Read the model definition and answer for the solid it produces. Units are mm, in the model's axes. Coordinates: 2 decimals unless noted, no trailing zeros. Loops run counter-clockwise (first coordinate to the right, second up) from the corner with the lowest first, then second, coordinate; pieces in that order, holes last. Notation, with made-up numbers: (29.25, -8) -> (70.25, -8) arc R23 cw to (70.25, 1) -> close; hole circle Ø9 at (50, 69.25). An arc over 180 degrees is marked (long way). Answer as a JSON object with one key per item and string values. Group by question number.
1) Section B-B, the plane y = 0 is taken. Give the vertices of the cut face in (x, z), plus the area to 3 significant figures.
2) Section D-D, the plane y = -37.7 is taken. Give the vertices of the cut face in (x, z).
3) Consider probe 1 along X at (y, z) = (0.5, 8.75); probe 2 along Y at (x, z) = (0, 7.25); probe 3 along Y at (x, z) = (17, 2.75). Determine where each line is inside the solid, lowest interval first. Write a range as [from, to].
4) Section A-A, the plane z = 8 is taken. Count the separate pieces of the cut face and the enclosed holes in it, plus the area to 3 significant figures.
5) Determine the mould class of faces 1 (the face through (36.325, -18.426, 4.93)), 2 (the face through (31.4, -18.8, 5.1)), 3 (the face through (-1, 1, 0)) for opening direction Y: released by +Y, released by -Y, zero draft, split by the parting line, or undercut.
6) Flat-ended cylindrical pins translate along their axes: P1, Ø3, axis at y = 10.5, z = 7, coming from the +X side; P2, Ø0.5, axis at x = 38.5, z = 3.5, coming from the -Y side; P3, Ø1.5, axis at y = -23.5, z = 6.5, coming from the -X side; P4, Ø2, axis at x = -32.65, y = -18.85, coming from the +Z side. Find the tip coordinate at first contact, or state that the pin passes through.
7) Section C-C, the plane x = 15 is taken. Give the vertices of the cut face in (y, z).
from build123d import *

# Parameters (mm, degrees)
SKETCH_1_R          = 45.3
EXTRUDE_1_DEPTH     = 10
CUT_EXTRUDE_1_DEPTH = 11
FILLET_1_R          = 3
SKETCH_3_R          = 1.25
CUT_EXTRUDE_2_DEPTH = 11
SKETCH_4_R          = 5.1
CUT_EXTRUDE_3_DEPTH = 11


with BuildPart() as part:
    # 草图1 → 凸台-拉伸1 (new body)
    with BuildSketch(Plane.XY):
        Circle(SKETCH_1_R)
    extrude(amount=EXTRUDE_1_DEPTH)

    # 草图2 → 切除-拉伸1 (cut, through all)
    with BuildSketch(Plane.XY.offset(10)):
        with BuildLine():
            Line((-36.056760808, 18), (-41.570301899, 18))
            ThreePointArc((-41.570301899, 18), (0, 45.3), (41.570301899, 18))
            Line((41.570301899, 18), (36.056760808, 18))
            ThreePointArc((36.056760808, 18), (0, 40.3), (-36.056760808, 18))
        make_face()
        with BuildLine():
            Line((-36.056760808, -18), (-41.734622438, -18))
            ThreePointArc((-41.734622438, -18), (0, -45.450838386), (41.734622438, -18))
            Line((41.734622438, -18), (36.056760808, -18))
            ThreePointArc((36.056760808, -18), (0, -40.3), (-36.056760808, -18))
        make_face()
    extrude(amount=-CUT_EXTRUDE_1_DEPTH, mode=Mode.SUBTRACT)

    # 圆角1
    fillet_1_edges = [part.edges().sort_by_distance(p)[0] for p in [
        (36.056760808, 18, 5),
        (-36.056760808, 18, 5),
        (-41.570301899, 18, 5),
        (41.570301899, 18, 5),
        (41.570301899, -18, 5),
        (36.056760808, -18, 5),
        (-41.570301899, -18, 5),
        (-36.056760808, -18, 5),
    ]]
    fillet(fillet_1_edges, radius=FILLET_1_R)

    # 草图3 → 切除-拉伸2 (cut, through all)
    with BuildSketch(Plane.XY.offset(10)):
        with Locations((0, 37.7)):
            Circle(SKETCH_3_R)
        with Locations((32.649157723, 18.85)):
            Circle(SKETCH_3_R)
        with Locations((32.649157723, -18.85)):
            Circle(SKETCH_3_R)
        with Locations((0, -37.7)):
            Circle(SKETCH_3_R)
        with Locations((-32.649157723, -18.85)):
            Circle(SKETCH_3_R)
        with Locations((-32.649157723, 18.85)):
            Circle(SKETCH_3_R)
    extrude(amount=-CUT_EXTRUDE_2_DEPTH, mode=Mode.SUBTRACT)

    # 草图4 → 切除-拉伸3 (cut, through all)
    with BuildSketch(Plane.XY.offset(10)):
        with Locations((-15, 0)):
            Circle(SKETCH_4_R)
        with Locations((15, 0)):
            Circle(SKETCH_4_R)
    extrude(amount=-CUT_EXTRUDE_3_DEPTH, mode=Mode.SUBTRACT)


solid = part.part
Determined:
{
 "1": {"outline": "(-45.3, 0) -> (-20.1, 0) -> (-20.1, 10) -> (-45.3, 10) -> close; (-9.9, 0) -> (9.9, 0) -> (9.9, 10) -> (-9.9, 10) -> close; (20.1, 0) -> (45.3, 0) -> (45.3, 10) -> (20.1, 10) -> close", "area": "702 mm²"},
 "2": {"outline": "(-14.24, 0) -> (-1.25, 0) -> (-1.25, 10) -> (-14.24, 10) -> close; (1.25, 0) -> (14.24, 0) -> (14.24, 10) -> (1.25, 10) -> close"},
 "3": {"probe 1": "[-45.3, -20.08], [-9.92, 9.92], [20.08, 45.3]", "probe 2": "[-40.3, -38.95], [-36.45, 36.45], [38.95, 40.3]", "probe 3": "[-36.54, -4.69], [4.69, 36.54]"},
 "4": {"separate pieces": "1", "enclosed holes": "8", "area": "5,280 mm²"},
 "5": {"face 1": "released by -Y", "face 2": "undercut", "face 3": "zero draft"},
 "6": {"P1": "x = 44.4", "P2": "y = -18", "P3": "x = -33.26", "P4": "through"},
 "7": {"outline": "(-37.4, 0) -> (-5.1, 0) -> (-5.1, 10) -> (-37.4, 10) -> close; (5.1, 0) -> (37.4, 0) -> (37.4, 10) -> (5.1, 10) -> close"}
}
